from build123d import *

# Parameters (mm, degrees)
F0_W     = 100
F0_H     = 50
F1_DEPTH = 3
F2_W     = 100
F2_H     = 50
F3_DEPTH = 3


with BuildPart() as f1:
    # F0 (on Front) → F1 (new body)
    with BuildSketch(Plane.XZ):
        Rectangle(F0_W, F0_H)
    extrude(amount=F1_DEPTH)

    # F2 (on Top) → F3 (join)
    with BuildSketch(Plane.XY):
        with Locations((-47.80928, 24.052748)):
            Rectangle(F2_W, F2_H)
    extrude(amount=F3_DEPTH)


solid = f1.part
Work out the finished part from the listing and answer in its coordinate system (mm). A direction names the side the tool comes from. Round coordinates to 2 decimals unless told otherwise and drop trailing zeros. Write each loop counter-clockwise with the first axis right and the second up, starting at its lowest first coordinate (ties: lowest second). Pieces come first, ordered by that corner, then holes.
1) Given pin 1 Ø2.5 at (x, z) = (-65, 2) entering from -Y; pin 2 Ø10 at (x, y) = (-29, 21.5) entering from -Z; pin 3 Ø4 at (x, z) = (-47, -14) entering from +Y; pin 4 Ø1.5 at (y, z) = (-1, 3.5) entering from -X, each flat-ended and moving along its own axis, determine where each tip first touches the part or whether it passes through.
2) A cutting plane is placed at A-A (x = -39.5). Give the vertices of the cut face in (y, z).
3) A tool of negligible diameter and unlimited length cuts with its end or side. For faces 1 (the flat face through (-74, -0.947, 1)), 2 (the flat face through (2.191, 24, 1)), 3 (the flat face through (-1, -1, 25)), from which of +Z, -Z, +X, -X, +Y, -Y can it reach the whole face along a straight path? Write none if from no direction.
4) A cutting plane is placed at B-B (z = -20). Give the vertices of the cut face in (x, y), plus the area to 3 significant figures.
5) Straight lines are drawn through the part: line 1 (Z direction, x = -23, y = 37); line 2 (Y direction, x = 42, z = -21); line 3 (X direction, y = 22.5, z = 2). For each, find the intervals that lie inside material, in ascending order.
6) A cutting plane is placed at C-C (y = 38). Give the vertices of the cut face in (x, z), plus the area to 3 significant figures.
Completed:
1. pin 1: stops at y = -0.95
1. pin 2: stops at z = 0
1. pin 3: stops at y = 0
1. pin 4: stops at x = -97.81
2. outline: (-3, -25) - (0, -25) - (0, 0) - (49.05, 0) - (49.05, 3) - (0, 3) - (0, 25) - (-3, 25) - close
3. face 1: +Z, -Z, -X, -Y
3. face 2: +Z, -Z, +X, +Y
3. face 3: +Z, +X, -X, +Y, -Y
4. outline: (-50, -3) - (50, -3) - (50, 0) - (-50, 0) - close
4. area: 300 mm2
5. line 1: z = 0 to 3
5. line 2: y = -3 to 0
5. line 3: x = -97.81 to 2.19
6. outline: (-97.81, 0) - (2.19, 0) - (2.19, 3) - (-97.81, 3) - close
6. area: 300 mm2
